from build123d import *

# Parameters (mm, degrees)
F0_W     = 15
F0_H     = 15
F1_DEPTH = 35
F2_W     = 3
F2_H     = 15
F3_DEPTH = 15
F4_R     = 1.5
F5_W     = 21.0236056261
F5_H     = 15
F6_DEPTH = 2.5
F7_R     = 0.5
F8_W     = 10.7259307988
F8_H     = 30.2171390504
F9_DEPTH = 25
F10_R    = 0.5
F11_R    = 0.5


with BuildPart() as f1:
    # F0 (on Top) → F1 (new body)
    with BuildSketch(Plane.XY):
        with Locations((0.8728443645, -1.2607762389)):
            Rectangle(F0_W, F0_H)
    extrude(amount=F1_DEPTH)

    # F2 (on face) → F3 (join, symmetric)
    with BuildSketch(Plane.XY.offset(35)):
        with Locations((-8.1271556355, -1.2607762389)):
            Rectangle(F2_W, F2_H)
        with Locations((9.8728443645, -1.2607762389)):
            Rectangle(F2_W, F2_H)
    extrude(amount=F3_DEPTH, both=True)

    # F4
    f4_edges = [f1.edges().sort_by_distance(p)[0] for p in [
        (11.372844, -1.260776, 20),
    ]]
    fillet(f4_edges, radius=F4_R)

    # F5 (on face) → F6 (join)
    with BuildSketch(Plane.XY.offset(50)):
        with Locations((0.8846471775, -1.2607762389)):
            Rectangle(F5_W, F5_H)
    extrude(amount=F6_DEPTH)

    # F7
    f7_edges = [f1.edges().sort_by_distance(p)[0] for p in [
        (0.884647, 6.239224, 52.5),
        (-9.627156, -1.260776, 52.5),
        (0.884647, -8.760776, 52.5),
        (11.39645, -1.260776, 52.5),
        (-9.627156, 6.239224, 36.25),
        (-9.627156, -8.760776, 36.25),
        (11.372844, 6.239224, 35.75),
        (0.872844, 6.239224, 35),
        (8.372844, 6.239224, 42.5),
        (0.872844, 6.239224, 50),
        (-6.627156, 6.239224, 42.5),
        (-6.627156, -8.760776, 10),
        (-9.627156, -1.260776, 20),
        (-6.627156, 6.239224, 10),
        (-6.627156, -1.260776, 0),
        (8.372844, 6.239224, 10),
        (0.872844, 6.239224, 0),
        (11.372844, -8.760776, 35.75),
        (8.372844, -8.760776, 10),
        (8.372844, -1.260776, 0),
        (11.372844, -1.260776, 21.5),
    ]]
    fillet(f7_edges, radius=F7_R)

    # F8 (on face) → F9 (cut)
    with BuildSketch(Plane(origin=(0, 6.2392237611, 0), x_dir=(-1, 0, 0), z_dir=(0, 1, 0))):
        with Locations((-0.938487472, 17.1604724601)):
            Rectangle(F8_W, F8_H)
    extrude(amount=-F9_DEPTH, mode=Mode.SUBTRACT)

    # F10
    f10_edges = [f1.edges().sort_by_distance(p)[0] for p in [
        (6.301453, 6.239224, 17.160472),
        (6.301453, -8.760776, 17.160472),
        (0.938487, 6.239224, 2.051903),
        (6.301453, -1.260776, 2.051903),
        (0.938487, -8.760776, 32.269042),
        (-4.424478, -8.760776, 17.160472),
        (0.938487, -8.760776, 2.051903),
        (-6.127156, -8.760776, 10),
        (-6.127156, -1.510776, 0),
        (-4.424478, 6.239224, 17.160472),
        (0.938487, 6.239224, 32.269042),
    ]]
    fillet(f10_edges, radius=F10_R)

    # F11
    f11_edges = [f1.edges().sort_by_distance(p)[0] for p in [
        (0.872844, -8.760776, 50),
        (-6.627156, -8.760776, 42.5),
        (0.872844, -8.760776, 35),
        (8.372844, -8.760776, 42.5),
    ]]
    fillet(f11_edges, radius=F11_R)


solid = f1.part
Model file for the job. Use its own axes, mm. A direction names the side the tool comes from. Give positions to 0.01 mm unless a question says otherwise; leave off trailing zeros. Order: outer loops, then holes, each group sorted by start corner. A loop starts at its lowest first (then second) coordinate and runs counter-clockwise, first axis right, second up. Notation, with made-up numbers: M 54.5,-16.75 L 94.5,-16.75 A9 ccw 94.5,-10.75 Z; hole C 73,7 d11. An arc over 180 degrees is marked long. Write item = value, one per line.
Q1. Cut at A-A, the plane z = 29. List the corners of the cut face in (x, y), then the cut area to 3 significant figures.
Derived:
outline = M -9.63,-8.26 A0.5 ccw -9.13,-8.76 L -4.92,-8.76 A0.5 ccw -4.42,-8.26 L -4.42,5.74 A0.5 ccw -4.92,6.24 L -9.13,6.24 A0.5 ccw -9.63,5.74 Z; M 6.3,-8.26 A0.5 ccw 6.8,-8.76 L 10.87,-8.76 A0.5 ccw 11.37,-8.26 L 11.37,5.74 A0.5 ccw 10.87,6.24 L 6.8,6.24 A0.5 ccw 6.3,5.74 Z
area = 154 mm2
Q2. Cut at B-B, the plane y = -3. Count the separate pieces of the cut face and the enclosed holes in it, then the cut area to 3 significant figures.
Derived:
separate_pieces = 1
enclosed_holes = 2
area = 433 mm2
Q3. Cut at D-D, the plane z = 42.5. List the corners of the cut face in (x, y), then the cut area to 3 significant figures.
Derived:
outline = M -9.63,-8.26 A0.5 ccw -9.13,-8.76 L -7.13,-8.76 A0.5 ccw -6.63,-8.26 L -6.63,5.74 A0.5 ccw -7.13,6.24 L -9.13,6.24 A0.5 ccw -9.63,5.74 Z; M 8.37,-8.26 A0.5 ccw 8.87,-8.76 L 10.87,-8.76 A0.5 ccw 11.37,-8.26 L 11.37,5.74 A0.5 ccw 10.87,6.24 L 8.87,6.24 A0.5 ccw 8.37,5.74 Z
area = 89.6 mm2
Q4. Cut at C-C, the plane x = 5.25. List the corners of the cut face in (y, z), then the cut area to 3 significant figures.
Derived:
outline = M -8.76,0 L 5.74,0 A0.5 ccw 6.24,0.5 L 6.24,1.55 A0.5 ccw 5.74,2.05 L -8.26,2.05 A0.5 ccw -8.76,1.55 Z; M -8.76,32.77 A0.5 ccw -8.26,32.27 L 5.74,32.27 A0.5 ccw 6.24,32.77 L 6.24,34.5 A0.5 ccw 5.74,35 L -8.26,35 A0.5 ccw -8.76,34.5 Z; M -8.76,50.5 A0.5 ccw -8.26,50 L 5.74,50 A0.5 ccw 6.24,50.5 L 6.24,52 A0.5 ccw 5.74,52.5 L -8.26,52.5 A0.5 ccw -8.76,52 Z
area = 109 mm2
Q5. Tool access for faces 5 (the flat face through (1, -1, 52.5)), 6 (the flat face through (9, -1, 20)), 7 (the flat face through (-6.627, -1, 10)), 8 (the flat face through (0, 6.239, 34)), 9 (the flat face through (6.301, -1, 17)): list every direction of +Z, -Z, +X, -X, +Y, -Y with a clear straight run to the whole face (end or side of a thin tool).
Derived:
face_5 = +Z, +X, -X, +Y, -Y
face_6 = -Z, +X, +Y, -Y
face_7 = -Z, -X, +Y, -Y
face_8 = +Z, -Z, +X, -X, +Y
face_9 = +Y, -Y
Q6. Flat gauge pins, fed straight in: pin 1 (2 mm diameter, centred on y = 3.5, z = 13, fed in from +X); pin 2 (8 mm diameter, centred on x = -5.5, y = 1, fed in from -Z); pin 3 (0.9 mm diameter, centred on x = -8, y = 1, fed in from -Z); pin 4 (6 mm diameter, centred on x = 1, z = 9, fed in from -Y) (3 decimals). Where does each tip first touch, or does it go through?
Derived:
pin_1 = 8.37
pin_2 = 0
pin_3 = 20
pin_4 = through
Q7. Drill centre lines: line 1 (Z direction, x = 3.25, y = 2.5); line 2 (X direction, y = 0, z = 19); line 3 (X direction, y = -5.5, z = 46.5). Where is each one in solid material? Low to high. Write a range as [from, to].
Derived:
line_1 = [0, 2.05], [32.27, 35], [50, 52.5]
line_2 = [-6.63, -4.42], [6.3, 8.37]
line_3 = [-9.63, -6.63], [8.37, 11.37]
Q8. Two-plate mould, pull along Z, no slides. Class faces 1 (the flat face through (-9.627, -1, 36)), 2 (the flat face through (8.373, -1, 43)), 3 (the flat face through (1, -1, 35)), 4 (the flat face through (1, -1, 0)): pulls with the +Z half, pulls with the -Z half, needs draft (parallel to the pull), parting line crosses it, or undercut.
Derived:
face_1 = needs draft
face_2 = undercut
face_3 = undercut
face_4 = pulls with the -Z half
